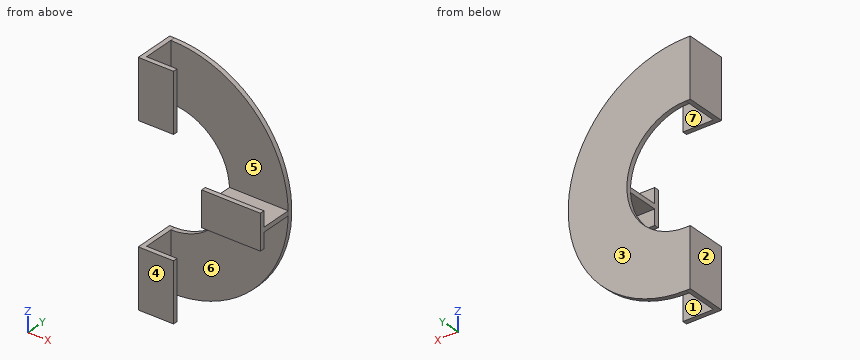
Autodesk Inventor part; units mm, degrees
ref_plane "YZ Plane" through (0, 0, 0) normal (1, 0, 0) x (0, 1, 0)
ref_plane "XZ Plane" through (0, 0, 0) normal (0, 1, 0) x (-1, 0, 0)
ref_plane "XY Plane" through (0, 0, 0) normal (0, 0, 1) x (1, 0, 0)
sketch "Sketch1" plane through (0, 0, 0) normal (0, 1, 0) x (-1, 0, 0)
  arc A0 (0, 100) -> (0, -100) centre (0, 0) ccw
  arc A1 (0, 200) -> (0, -200) centre (0, 0) ccw
  line L0 (0, 200) -> (0, 100)
  line L1 (0, -100) -> (0, -200)
  dimension "d0" = 200
  dimension "d1" = 400
extrude "Extrusion1" add sketch "Sketch1" along normal blind 8
sketch "Sketch2" plane through (0, 8, 0) normal (0, 1, 0) x (1, 0, 0)
  line L0 (0, -100) -> (0, -200)
  line L1 (0, -200) -> (-8, -200)
  line L2 (-8, -200) -> (-8, -100)
  line L3 (-8, -100) -> (0, -100)
  line L4 (0, -100) -> (0, -200)
  line L5 (0, 200) -> (0, 100)
  line L6 (0, 100) -> (0, 200)
  line L7 (0, 200) -> (-8, 200)
  line L8 (-8, 200) -> (-8, 100)
  line L9 (-8, 100) -> (0, 100)
  point P0 (0, 0)
  dimension "d4" = 8
  dimension "d5" = 100
  dimension "d6" = 8
  dimension "d7" = 100
extrude "Extrusion2" add sketch "Sketch2" against normal blind 62
sketch "Sketch3" plane through (0, -54, 0) normal (0, -1, 0) x (1, 0, 0)
  line L0 (-8, -100) -> (-8, -200)
  line L1 (-8, -200) -> (52, -200)
  line L2 (52, -200) -> (52, -100)
  line L3 (52, -100) -> (-8, -100)
  line L4 (-8, -100) -> (-8, -200)
  line L5 (-8, 200) -> (-8, 100)
  line L6 (-8, 100) -> (52, 100)
  line L7 (52, 100) -> (52, 200)
  line L8 (52, 200) -> (-8, 200)
  line L9 (-8, 200) -> (-8, 100)
  point P0 (0, 0)
  dimension "d10" = 60
  dimension "d11" = 60
extrude "Extrusion3" add sketch "Sketch3" along normal blind 8
sketch "Sketch4" plane through (0, 0, 0) normal (0, -1, 0) x (1, 0, 0)
  arc A0 (0, -100) -> (0, 100) centre (0, 0) ccw
  line L0 (100, 0) -> (200, 0)
  line L1 (200, 0) -> (200, 4)
  line L2 (200, 4) -> (100, 4)
  line L3 (100, 4) -> (100, 0)
  line L4 (100, 0) -> (200, 0)
  line L5 (200, 0) -> (200, -4)
  line L6 (200, -4) -> (100, -4)
  line L7 (100, -4) -> (100, 0)
  dimension "d14" = 100
  dimension "d15" = 4
  dimension "d16" = 100
  dimension "d17" = 4
extrude "Extrusion4" add sketch "Sketch4" along normal blind 54
sketch "Sketch5" plane through (0, -54, 0) normal (0, -1, 0) x (1, 0, 0)
  line L0 (200, -4) -> (200, 4)
  line L1 (200, 0) -> (100, 0)
  line L2 (100, 0) -> (100, -30)
  line L3 (100, -30) -> (200, -30)
  line L4 (200, -30) -> (200, 0)
  line L5 (200, 0) -> (100, 0)
  line L6 (100, 0) -> (100, 30)
  line L7 (100, 30) -> (200, 30)
  line L8 (200, 30) -> (200, 0)
  point P0 (0, 0)
  dimension "d20" = 100
  dimension "d21" = 30
  dimension "d22" = 100
  dimension "d23" = 30
extrude "Extrusion5" add sketch "Sketch5" along normal blind 8
sketch "Sketch6" plane through (0, 8, 0) normal (0, 1, 0) x (1, 0, 0)
  circle A0 centre (146.0864, 0) radius 2.5
  point P0 (0, 0)
  dimension "d26" = 5
properties part number "Cuptable1" material "Wood (Birch)"
The model under review builds one solid part; all positions refer to its coordinate system, in mm. Face numbers are marked on the shaded views. A direction names the side the tool comes from. Round coordinates to 2 decimals unless told otherwise and drop trailing zeros. Write each loop counter-clockwise with the first axis right and the second up, starting at its lowest first coordinate (ties: lowest second). Pieces come first, ordered by that corner, then holes. Notation, with made-up numbers: M -5,20.5 L 45,20.5 A23 ccw 45,48.5 Z; hole C 85,-40 d6. An arc over 180 degrees is marked long. Use CSV: the item, a comma, the result in double quotes. Start each with the question number.
(1) Clearance check with flat-ended pins moving along their axes: P1, Ø18, axis at y = -38.5, z = -14.5, coming from the -X side; P2, Ø16, axis at y = -30, z = -167, coming from the +X side; P3, Ø4, axis at x = 151, y = -59.5, coming from the +Z side; P4, Ø9, axis at y = -58, z = 151.5, coming from the +X side. State where each tip first meets the part, or that it passes through.
(2) Tool access review of the marked faces 4, 5, 6 and 7: name each direction out of +Z, -Z, +X, -X, +Y, -Y from which nothing blocks a thin tool from reaching the whole face with its end or side.
(3) We need section B-B, the plane x = 33. State the section outline as (y, z) points, then the cut area to 3 significant figures.
(4) We need section C-C, the plane z = 150. State the section outline as (x, y) points, then the cut area to 3 significant figures.
(5) The part is to be moulded in two halves that separate along Y. For the marked faces 1, 2 and 3, say which applies: +Y half, -Y half, draft (parallel to the pull), parting line (faces both ways), or undercut.
(6) We need section A-A, the plane y = -4. State the section outline as (x, z) points, then the cut area to 3 significant figures.
(7) We need section D-D, the plane x = 149.5. State the section outline as (y, z) points.
(8) For line 1 along Y through (x, z) = (50.5, -162.5); line 2 along Y through (x, z) = (121.5, 94); line 3 along Z through (x, y) = (114, -1), list the stretches that pass through material, from the lowest coordinate up.
Findings:
1,P1,"through"
1,P2,"x = 0"
1,P3,"z = 30"
1,P4,"x = 52"
2,face 4,"+Z, -Z, +X, -X, -Y"
2,face 5,"+Z, +X"
2,face 6,"-Z, +X"
2,face 7,"+Z, -Z, +X"
3,outline,"M -62,-200 L -54,-200 L -54,-100 L -62,-100 Z; M -62,100 L -54,100 L -54,200 L -62,200 Z; M 0,-197.26 L 8,-197.26 L 8,-94.4 L 0,-94.4 Z; M 0,94.4 L 8,94.4 L 8,197.26 L 0,197.26 Z"
3,area,"3,250 mm^2"
4,outline,"M -8,-62 L 52,-62 L 52,-54 L 0,-54 L 0,0 L 132.29,0 L 132.29,8 L -8,8 Z"
4,area,"2,030 mm^2"
5,face 1,"undercut"
5,face 2,"draft"
5,face 3,"+Y half"
6,outline,"M -8,-200 L 0,-200 L 0,-100 L -8,-100 Z; M -8,100 L 0,100 L 0,200 L -8,200 Z; M 100,-4 L 200,-4 L 200,4 L 100,4 Z"
6,area,"2,400 mm^2"
7,outline,"M -62,-30 L -54,-30 L -54,-4 L 0,-4 L 0,-132.85 L 8,-132.85 L 8,132.85 L 0,132.85 L 0,4 L -54,4 L -54,30 L -62,30 Z"
8,line 1,"-62 to -54, 0 to 8"
8,line 2,"0 to 8"
8,line 3,"-4 to 4"
